Answer from the drawing. Dimensions are ordinates in mm from the lowest x, y and z of the part. A direction names the side the tool comes from. Give positions to 0.01 mm unless a question says otherwise; leave off trailing zeros. Write each loop counter-clockwise with the first axis right and the second up, starting at its lowest first coordinate (ties: lowest second). Pieces come first, ordered by that corner, then holes. Notation, with made-up numbers: M 8.25,-37.5 L 57.25,-37.5 A30 ccw 57.25,-3.5 Z; hole C -31.75,8 d11. An arc over 180 degrees is marked long. Answer as a JSON object with one key per item and string values.
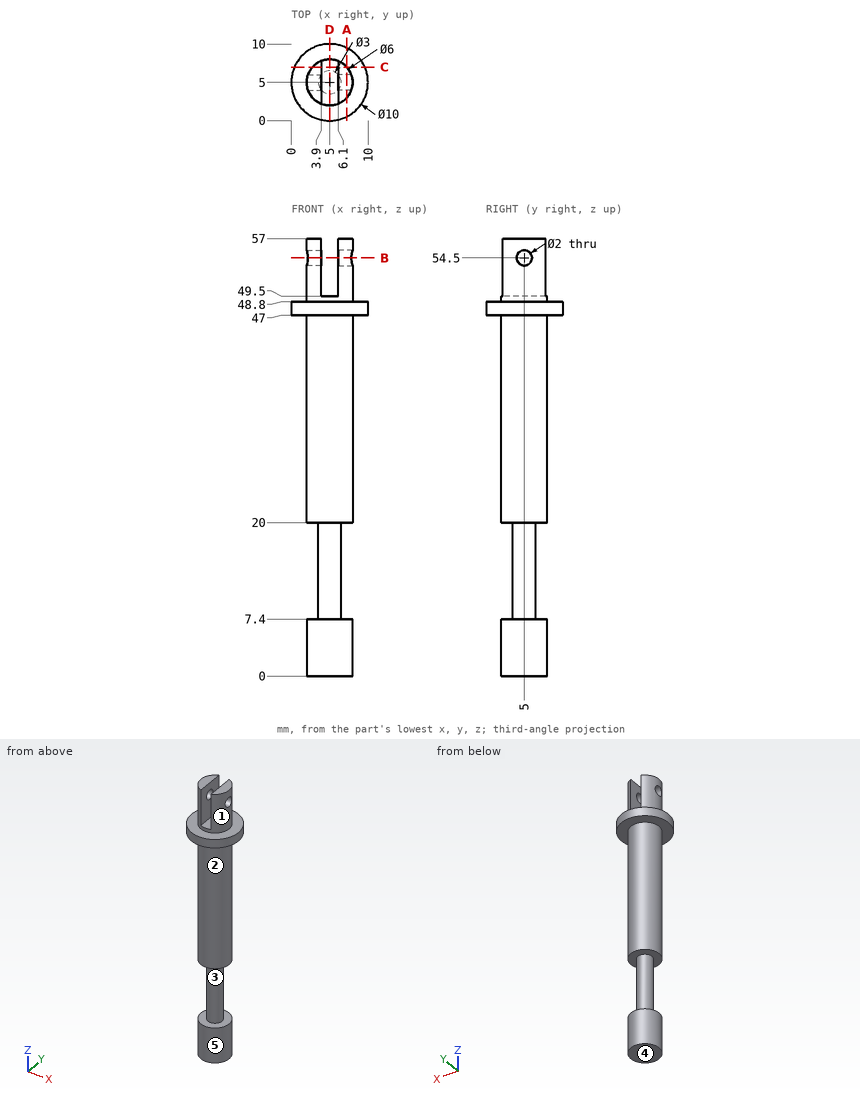
1. A cutting plane is placed at C-C, the plane y = 7. Give the vertices of the cut face in (x, z), plus the area to 3 significant figures.
Verdict:
{"outline": "M 0.42,47 L 2.76,47 L 2.76,20 L 7.24,20 L 7.24,47 L 9.58,47 L 9.58,48.8 L 7.24,48.8 L 7.24,57 L 6.1,57 L 6.1,49.5 L 3.9,49.5 L 3.9,57 L 2.76,57 L 2.76,48.8 L 0.42,48.8 Z; M 2.76,0 L 7.24,0 L 7.24,7.4 L 2.76,7.4 Z", "area": "191 mm2"}
2. A cutting plane is placed at D-D, the plane x = 5. Give the vertices of the cut face in (y, z), plus the area to 3 significant figures.
Verdict:
{"outline": "M 0,47 L 2,47 L 2,20 L 3.5,20 L 3.5,7.4 L 2,7.4 L 2,0 L 8,0 L 8,7.4 L 6.5,7.4 L 6.5,20 L 8,20 L 8,47 L 10,47 L 10,48.8 L 8,48.8 L 8,49.5 L 2,49.5 L 2,48.8 L 0,48.8 Z", "area": "266 mm2"}
3. A cutting plane is placed at A-A, the plane x = 7.25. Give the vertices of the cut face in (y, z), plus the area to 3 significant figures.
Verdict:
{"outline": "M 0.53,47 L 3.02,47 L 3.02,20 L 6.98,20 L 6.98,47 L 9.47,47 L 9.47,48.8 L 6.98,48.8 L 6.98,57 L 3.02,57 L 3.02,48.8 L 0.53,48.8 Z; M 3.02,0 L 6.98,0 L 6.98,7.4 L 3.02,7.4 Z; hole C 5,54.5 d2", "area": "182 mm2"}
4. Consider line 1 along Z through (x, y) = (6.6, 5); line 2 along Z through (x, y) = (0.5, 5.75); line 3 along Y through (x, z) = (2.8, 54.5). Determine where each line is inside the solid, lowest interval first.
Verdict:
{"line 1": "z = 0 to 7.4, 20 to 53.5, 55.5 to 57", "line 2": "z = 47 to 48.8", "line 3": "y = 2.96 to 4, 6 to 7.04"}
5. The mould has two halves that part along Z. Classify the marked faces 3, 4 and 5: released by +Z, released by -Z, zero draft, split by the parting line, or undercut.
Verdict:
{"face 3": "undercut", "face 4": "released by -Z", "face 5": "zero draft"}
6. For the marked faces 1 and 2, determine the directions among +Z, -Z, +X, -X, +Y, -Y from which every point of the face is accessible in a straight line to the end or side of a thin tool.
Verdict:
{"face 1": "+Z", "face 2": "-Z"}
7. A cutting plane is placed at B-B, the plane z = 54.5. Give the vertices of the cut face in (x, y), plus the area to 3 significant figures.
Verdict:
{"outline": "M 2.17,4 A3 ccw 3.9,2.21 L 3.9,4 Z; M 2.17,6 L 3.9,6 L 3.9,7.79 A3 ccw Z; M 6.1,2.21 A3 ccw 7.83,4 L 6.1,4 Z; M 6.1,6 L 7.83,6 A3 ccw 6.1,7.79 Z", "area": "8.00 mm2"}
8. Flat-ended cylindrical pins translate along their axes: pin 1 (1 mm diameter, centred on y = 8, z = 14, fed in from +X); pin 2 (1.1 mm diameter, centred on x = 4.5, y = 6, fed in from +Z); pin 3 (1.7 mm diameter, centred on y = 6, z = 53.5, fed in from -X); pin 4 (1 mm diameter, centred on y = 3, z = 7.5, fed in from +X). Find the tip coordinate at first contact, or state that the pin passes through.
Verdict:
{"pin 1": "passes through", "pin 2": "stops at z = 49.5", "pin 3": "stops at x = 2", "pin 4": "stops at x = 7.59"}
